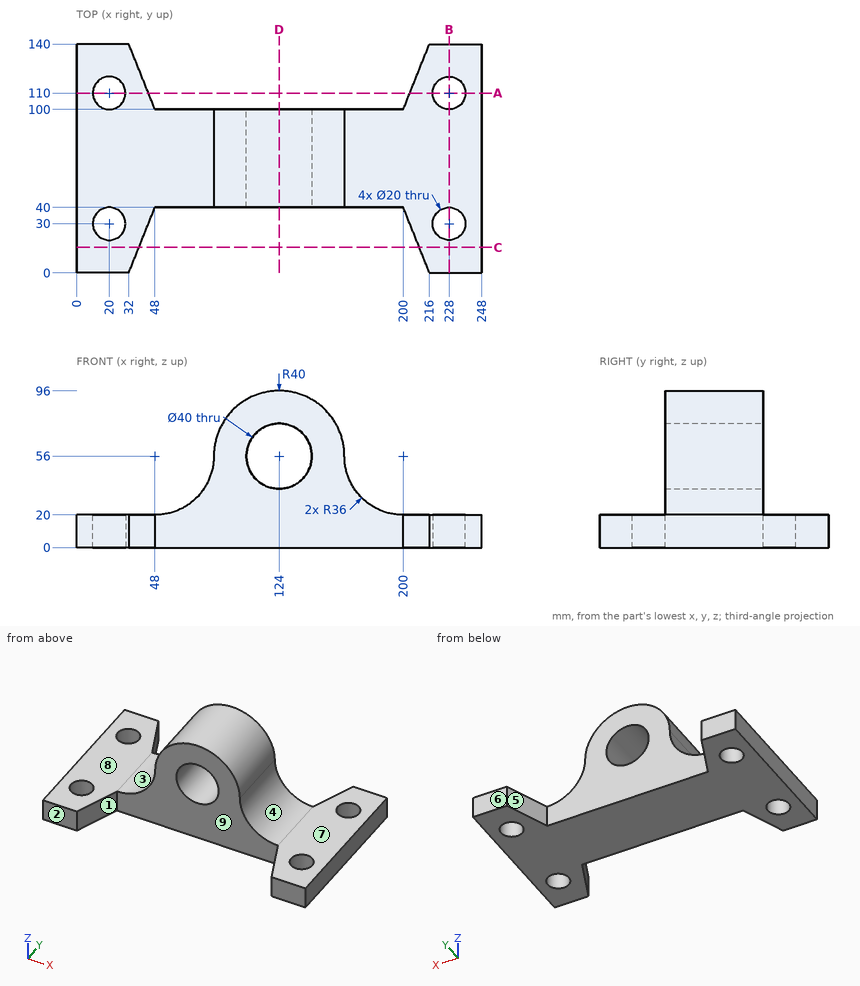
Geometry check sheet. Reference: drawing and pictorial views, mm from the part's lowest x, y, z. A direction names the side the tool comes from. Coordinates: 2 decimals unless noted, no trailing zeros. Order: outer loops, then holes, each group sorted by start corner. A loop starts at its lowest first (then second) coordinate and runs counter-clockwise, first axis right, second up. Notation, with made-up numbers: (56.5, -31.75) -> (64.5, -31.75) arc R17 ccw to (64.5, -23.75) -> close; hole circle Ø6 at (33, 40.5). An arc over 180 degrees is marked (long way). Use CSV: the item, a comma, the result in double quotes. Start each with the question number.
Q1. Section check B-B, the plane x = 228. Record the cut outline in (y, z).
Q2. Tool access check on the marked faces 5, 6, 7, 8 and 9. Record the directions out of +Z, -Z, +X, -X, +Y, -Y that give a thin tool (end or side, any length) a straight path to the whole face; none if there is none.
Q3. Section check C-C, the plane y = 15.5. Record the cut outline in (x, z), and give its area (3 significant figures).
Q4. Draft check along X on the marked faces 1, 2, 3 and 4. Enter one of: +X half, -X half, draft (parallel to the pull), parting line (faces both ways), or undercut.
Q5. Thickness scan on line 1 along Y through (x, z) = (20, 7.5); line 2 along Y through (x, z) = (229, 6.5); line 3 along Z through (x, y) = (124, 81.5). Record the ranges inside material, lowest first.
Q6. Depth check by flat-ended pin: P1, Ø18, axis at x = 228, y = 110, coming from the +Z side; P2, Ø14.5, axis at x = 222.5, y = 62, coming from the +Z side; P3, Ø1, axis at x = 44, z = 12, coming from the -Y side. Enter the tip coordinate at first touch or a pass-through.
Q7. Section check D-D, the plane x = 124. Record the cut outline in (y, z), and give its area (3 significant figures).
Q8. Section check A-A, the plane y = 110. Record the cut outline in (x, z).
Returned:
1,outline,"(0, 0) -> (20, 0) -> (20, 20) -> (0, 20) -> close; (40, 0) -> (100, 0) -> (100, 20) -> (40, 20) -> close; (120, 0) -> (140, 0) -> (140, 20) -> (120, 20) -> close"
2,face 5,"+Z, -Z, +Y"
2,face 6,"+Z, -Z, +X, -X, +Y"
2,face 7,"+Z, +X, +Y, -Y"
2,face 8,"+Z, -X, +Y, -Y"
2,face 9,"+Z, -Z, -Y"
3,outline,"(0, 0) -> (38.2, 0) -> (38.2, 20) -> (0, 20) -> close; (209.8, 0) -> (248, 0) -> (248, 20) -> (209.8, 20) -> close"
3,area,"1,530 mm^2"
4,face 1,"undercut"
4,face 2,"draft"
4,face 3,"-X half"
4,face 4,"+X half"
5,line 1,"y = 0 to 20, 40 to 100, 120 to 140"
5,line 2,"y = 0 to 20.05, 39.95 to 100.05, 119.95 to 140"
5,line 3,"z = 0 to 36, 76 to 96"
6,P1,"passes through"
6,P2,"stops at z = 20"
6,P3,"stops at y = 28.75"
7,outline,"(40, 0) -> (100, 0) -> (100, 36) -> (40, 36) -> close; (40, 76) -> (100, 76) -> (100, 96) -> (40, 96) -> close"
7,area,"3,360 mm^2"
8,outline,"(0, 0) -> (10, 0) -> (10, 20) -> (0, 20) -> close; (30, 0) -> (44, 0) -> (44, 20) -> (30, 20) -> close; (204, 0) -> (218, 0) -> (218, 20) -> (204, 20) -> close; (238, 0) -> (248, 0) -> (248, 20) -> (238, 20) -> close"
